Input: part model. Units: mm. Frame: model coordinates. Face numbers are marked on the shaded views. A direction names the side the tool comes from. Coordinates: 2 decimals unless noted, no trailing zeros. Write each loop counter-clockwise with the first axis right and the second up, starting at its lowest first coordinate (ties: lowest second). Pieces come first, ordered by that corner, then holes. Notation, with made-up numbers: M 72,-10.75 L 129,-10.75 A18 ccw 129,16.25 Z; hole C 67.25,-4.5 d4. An arc over 180 degrees is marked long. Use one line per item in the form item = value.
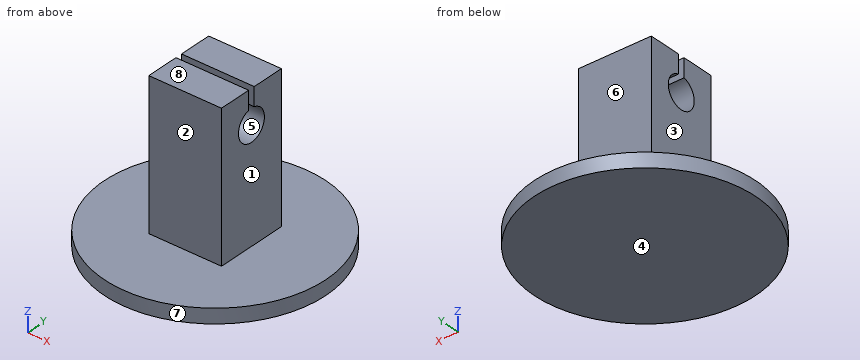
from build123d import *

# Parameters (mm, degrees)
F0_R     = 22.8354
F1_DEPTH = 3
F2_W     = 15
F2_H     = 15
F3_DEPTH = 30
F5_DEPTH = 25


with BuildPart() as f1:
    # F0 (on Top) → F1 (new body)
    with BuildSketch(Plane.XY):
        Circle(F0_R)
    extrude(amount=F1_DEPTH)

    # F2 (on face) → F3 (join)
    with BuildSketch(Plane.XY.offset(3)):
        Rectangle(F2_W, F2_H)
    extrude(amount=F3_DEPTH)

    # F4 (on face) → F5 (cut)
    with BuildSketch(Plane(origin=(-7.5, 0, 0), x_dir=(0, -1, 0), z_dir=(-1, 0, 0))):
        with BuildLine():
            Line((-0.7, 33), (-0.7, 29.17372))
            ThreePointArc((-0.7, 29.17372), (0, 22.75), (0.7, 29.17372))
            Line((0.7, 29.17372), (0.7, 33))
            Line((0.7, 33), (-0.7, 33))
        make_face()
    extrude(amount=-F5_DEPTH, mode=Mode.SUBTRACT)


solid = f1.part
(1) Section query B-B on y = 0. Return the cut outline in (x, z).
Computed:
outline = M -22.84,0 L 22.84,0 L 22.84,3 L 7.5,3 L 7.5,22.75 L -7.5,22.75 L -7.5,3 L -22.84,3 Z
(2) Section query C-C on x = 0. Return the cut outline in (y, z), plus the area to 3 significant figures.
Computed:
outline = M -22.84,0 L 22.84,0 L 22.84,3 L 7.5,3 L 7.5,33 L 0.7,33 L 0.7,29.17 A3.25 cw long -0.7,29.17 L -0.7,33 L -7.5,33 L -7.5,3 L -22.84,3 Z
area = 549 mm^2
(3) First-contact query: pin 1 Ø8 at (x, y) = (14, 7) entering from -Z; pin 2 Ø4 at (x, z) = (-2.5, 31.5) entering from -Y; pin 3 Ø10 at (x, z) = (9.5, 13.5) entering from +Y; pin 4 Ø7.5 at (y, z) = (-2.5, 24) entering from -X. Flat tips, straight axial feed; report the tip coordinate or a pass-through.
Computed:
pin_1 = 0
pin_2 = -7.5
pin_3 = 7.5
pin_4 = -7.5
(4) Section query A-A on z = 26. Return the cut outline in (x, y), plus the area to 4 significant figures.
Computed:
outline = M -7.5,-7.5 L 7.5,-7.5 L 7.5,-3.25 L -7.5,-3.25 Z; M -7.5,3.25 L 7.5,3.25 L 7.5,7.5 L -7.5,7.5 Z
area = 127.5 mm^2
(5) Pull-direction query (Y, two-part tool) for the marked faces 5, 6, 7 and 8; classes: pulls with the +Y half, pulls with the -Y half, needs draft (parallel to the pull), parting line crosses it, or undercut.
Computed:
face_5 = undercut
face_6 = pulls with the +Y half
face_7 = parting line crosses it
face_8 = needs draft
(6) Set-up query: the marked faces 1, 2, 3 and 4. Return all of +Z, -Z, +X, -X, +Y, -Y with unobstructed straight access to the full face (end or side cutting, diameter ignored); none if empty.
Computed:
face_1 = +Z, +X, +Y, -Y
face_2 = +Z, +X, -X, -Y
face_3 = +Z, -X, +Y, -Y
face_4 = -Z, +X, -X, +Y, -Y
(7) Section query D-D on z = 21. Return the cut outline in (x, y), plus the area to 3 significant figures.
Computed:
outline = M -7.5,-7.5 L 7.5,-7.5 L 7.5,7.5 L -7.5,7.5 Z
area = 225 mm^2
(8) Line query: probe 1 along Y at (x, z) = (4, 31); probe 2 along Y at (x, z) = (0, 26); probe 3 along Z at (x, y) = (11.5, -13). Output: solid intervals per line, ascending.
Computed:
probe_1 = -7.5 to -0.7, 0.7 to 7.5
probe_2 = -7.5 to -3.25, 3.25 to 7.5
probe_3 = 0 to 3
